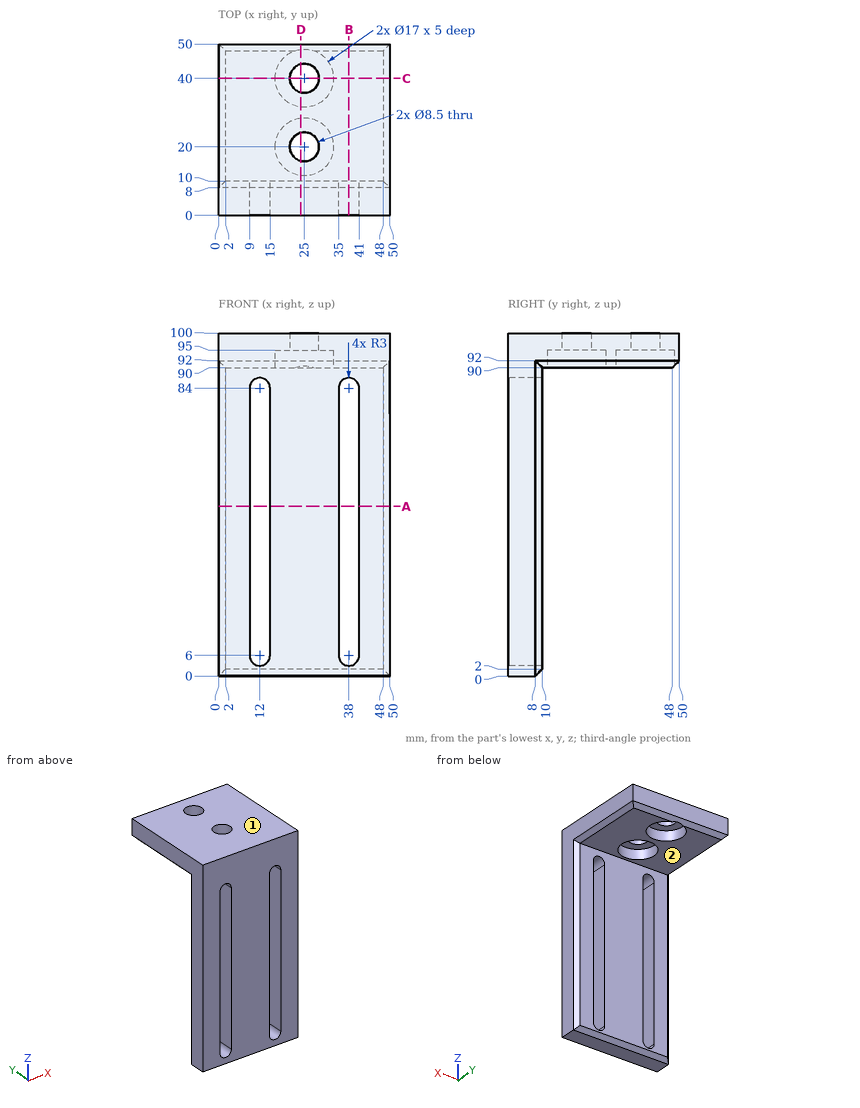
Drawing for the job (mm, zero at the part's lowest x, y, z). A direction names the side the tool comes from. Round coordinates to 2 decimals unless told otherwise and drop trailing zeros. Write each loop counter-clockwise with the first axis right and the second up, starting at its lowest first coordinate (ties: lowest second). Pieces come first, ordered by that corner, then holes.
Item 1: Band-saw the part on C-C on y = 40. Write the cut outline in (x, z), then the cut area to 4 significant figures.
Filled in:
outline: (0, 92) - (2, 90) - (16.5, 90) - (16.5, 95) - (20.75, 95) - (20.75, 100) - (0, 100) - close; (29.25, 95) - (33.5, 95) - (33.5, 90) - (48, 90) - (50, 92) - (50, 100) - (29.25, 100) - close
area: 368.5 mm2
Item 2: Drop flat-ended pins along their axis: pin 1 Ø11.5 at (x, y) = (20, 36.5) entering from -Z; pin 2 Ø8.5 at (x, y) = (25, 42) entering from -Z; pin 3 Ø4 at (x, z) = (9.5, 51.5) entering from +Y. Give the stop position or say it passes through.
Filled in:
pin 1: stops at z = 90
pin 2: stops at z = 95
pin 3: stops at y = 10
Item 3: Band-saw the part on A-A on z = 49.5. Write the cut outline in (x, y), then the cut area to 3 significant figures.
Filled in:
outline: (0, 0) - (9, 0) - (9, 10) - (2, 10) - (0, 8) - close; (15, 0) - (35, 0) - (35, 10) - (15, 10) - close; (41, 0) - (50, 0) - (50, 8) - (48, 10) - (41, 10) - close
area: 376 mm2
Item 4: Drill centre lines: L1, parallel to X at y = 3, z = 15; L2, parallel to Y at x = 25, z = 98.85; L3, parallel to Y at x = 25, z = 92. Where is each one in solid material? Low to high.
Filled in:
L1: x = 0 to 9, 15 to 35, 41 to 50
L2: y = 0 to 15.75, 24.25 to 35.75, 44.25 to 50
L3: y = 0 to 11.5, 28.5 to 31.5, 48.5 to 50
Item 5: Band-saw the part on B-B on x = 38. Write the cut outline in (y, z).
Filled in:
outline: (0, 0) - (8, 0) - (10, 2) - (10, 3) - (0, 3) - close; (0, 87) - (10, 87) - (10, 90) - (48, 90) - (50, 92) - (50, 100) - (0, 100) - close
Item 6: Band-saw the part on D-D on x = 24. Write the cut outline in (y, z), then the cut area to 3 significant figures.
Filled in:
outline: (0, 0) - (8, 0) - (10, 2) - (10, 90) - (11.56, 90) - (11.56, 95) - (15.87, 95) - (15.87, 100) - (0, 100) - close; (24.13, 95) - (28.44, 95) - (28.44, 90) - (31.56, 90) - (31.56, 95) - (35.87, 95) - (35.87, 100) - (24.13, 100) - close; (44.13, 95) - (48.44, 95) - (48.44, 90.44) - (50, 92) - (50, 100) - (44.13, 100) - close
area: 1,140 mm2
Item 7: Tool access for the marked faces 1 and 2: list every direction of +Z, -Z, +X, -X, +Y, -Y with a clear straight run to the whole face (end or side of a thin tool).
Filled in:
face 1: +Z, +X, -X, +Y, -Y
face 2: -Z, +X, -X, +Y
